Design review of the part built by this model. Coordinates are the model's own, in mm. Face numbers are marked on the shaded views. A direction names the side the tool comes from. Coordinates: 2 decimals unless noted, no trailing zeros. Order: outer loops, then holes, each group sorted by start corner. A loop starts at its lowest first (then second) coordinate and runs counter-clockwise, first axis right, second up. Notation, with made-up numbers: M -1.5,13 L 24.5,13 A30 cw 24.5,50 Z; hole C 22.25,37 d3. An arc over 180 degrees is marked long. Answer as a JSON object with one key per item and string values.
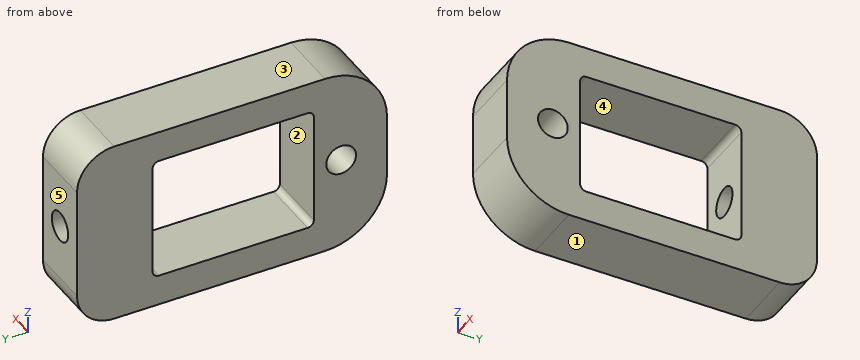
from build123d import *

# Parameters (mm, degrees)
SKETCH16_W                 = 5
SKETCH16_H                 = 15
MAIN_EXTRUDE_LOCKING_DEPTH = 25
SKETCH18_R                 = 1.2
CUT_EXTRUDE1_DEPTH         = 5
SKETCH8_W                  = 10
SKETCH8_H                  = 13
CUT_EXTRUDE2_DEPTH         = 5
SKETCH9_R                  = 1.2
CUT_EXTRUDE3_DEPTH         = 6.1
FILLET1_R                  = 5
FILLET2_R                  = 3
FILLET3_R                  = 0.5


with BuildPart() as part:
    # Sketch16 → Main Extrude_Locking (new body)
    with BuildSketch(Plane(origin=(0, 0, 0), x_dir=(1, 0, 0), z_dir=(0, 1, 0))):
        Rectangle(SKETCH16_W, SKETCH16_H)
    extrude(amount=MAIN_EXTRUDE_LOCKING_DEPTH)

    # Sketch18 → Cut-Extrude1 (cut)
    with BuildSketch(Plane.ZY.offset(2.5)):
        with Locations((0, 3.7)):
            Circle(SKETCH18_R)
    extrude(amount=-CUT_EXTRUDE1_DEPTH, mode=Mode.SUBTRACT)

    # Sketch8 → Cut-Extrude2 (cut)
    with BuildSketch(Plane.ZY.offset(2.5)):
        with Locations((0, 12.4)):
            Rectangle(SKETCH8_W, SKETCH8_H)
    extrude(amount=-CUT_EXTRUDE2_DEPTH, mode=Mode.SUBTRACT)

    # Sketch9 → Cut-Extrude3 (cut)
    with BuildSketch(Plane(origin=(0, 25, 0), x_dir=(1, 0, 0), z_dir=(0, 1, 0))):
        with Locations(Location((0, 0, 0), (0, 0, 270))):
            Circle(SKETCH9_R)
    extrude(amount=-CUT_EXTRUDE3_DEPTH, mode=Mode.SUBTRACT)

    # Fillet1
    fillet1_edges = [part.edges().sort_by_distance(p)[0] for p in [
        (0, 0, 7.5),
        (0, 0, -7.5),
    ]]
    fillet(fillet1_edges, radius=FILLET1_R)

    # Fillet2
    fillet2_edges = [part.edges().sort_by_distance(p)[0] for p in [
        (0, 25, 7.5),
        (0, 25, -7.5),
    ]]
    fillet(fillet2_edges, radius=FILLET2_R)

    # Fillet3
    fillet3_edges = [part.edges().sort_by_distance(p)[0] for p in [
        (0, 5.9, -5),
        (0, 18.9, -5),
        (0, 18.9, 5),
        (0, 5.9, 5),
    ]]
    fillet(fillet3_edges, radius=FILLET3_R)


solid = part.part
1) To check wall thickness, follow L1, parallel to Z at x = -0.1, y = 22; L2, parallel to Y at x = -0.2, z = 0; L3, parallel to Z at x = 2.1, y = 12.75. State the ranges of each line that lie inside material, in increasing order.
Taken from the geometry:
{"L1": "z = -7.5 to -1.2, 1.2 to 7.5", "L2": "y = 0 to 2.5, 4.9 to 5.9", "L3": "z = -7.5 to -5, 5 to 7.5"}
2) Add section A-A (y = 12). State the section outline as (x, z) points, and give its area (3 significant figures).
Taken from the geometry:
{"outline": "M -2.5,-7.5 L 2.5,-7.5 L 2.5,-5 L -2.5,-5 Z; M -2.5,5 L 2.5,5 L 2.5,7.5 L -2.5,7.5 Z", "area": "25.0 mm2"}
3) Add section C-C (x = 1.8). State the section outline as (y, z) points.
Taken from the geometry:
{"outline": "M 0,-2.5 A5 ccw 5,-7.5 L 22,-7.5 A3 ccw 25,-4.5 L 25,4.5 A3 ccw 22,7.5 L 5,7.5 A5 ccw 0,2.5 Z; hole C 3.7,0 d2.4; hole M 5.9,-4.5 A0.5 ccw 6.4,-5 L 18.4,-5 A0.5 ccw 18.9,-4.5 L 18.9,4.5 A0.5 ccw 18.4,5 L 6.4,5 A0.5 ccw 5.9,4.5 Z"}
4) Tool access review of the marked faces 4 and 5: name each direction out of +Z, -Z, +X, -X, +Y, -Y from which nothing blocks a thin tool from reaching the whole face with its end or side.
Taken from the geometry:
{"face 4": "+X, -X", "face 5": "+Z, -Z, +X, -X, +Y"}
5) Mouldability with a two-part tool opening along Z and no side actions: class the marked faces 1, 2 and 3 as released by +Z, released by -Z, zero draft, split by the parting line, or undercut.
Taken from the geometry:
{"face 1": "released by -Z", "face 2": "undercut", "face 3": "released by +Z"}
6) Add section B-B (z = 0). State the section outline as (x, y) points.
Taken from the geometry:
{"outline": "M -2.5,0 L 2.5,0 L 2.5,2.5 L -2.5,2.5 Z; M -2.5,4.9 L 2.5,4.9 L 2.5,5.9 L -2.5,5.9 Z; M -2.5,18.9 L -1.2,18.9 L -1.2,25 L -2.5,25 Z; M 1.2,18.9 L 2.5,18.9 L 2.5,25 L 1.2,25 Z"}
7) Add section D-D (x = 0). State the section outline as (y, z) points.
Taken from the geometry:
{"outline": "M 0,-2.5 A5 ccw 5,-7.5 L 22,-7.5 A3 ccw 25,-4.5 L 25,-1.2 L 18.9,-1.2 L 18.9,-4.5 A0.5 cw 18.4,-5 L 6.4,-5 A0.5 cw 5.9,-4.5 L 5.9,4.5 A0.5 cw 6.4,5 L 18.4,5 A0.5 cw 18.9,4.5 L 18.9,1.2 L 25,1.2 L 25,4.5 A3 ccw 22,7.5 L 5,7.5 A5 ccw 0,2.5 Z; hole C 3.7,0 d2.4"}
8) Insertion check: pin 1 Ø2 at (y, z) = (13.5, -4.5) entering from -X; pin 2 Ø1.9 at (y, z) = (3.7, 0) entering from +X. Each pin has a flat end and moves straight along its axis. Give the tip position at first contact, or say it passes through.
Taken from the geometry:
{"pin 1": "stops at x = -2.5", "pin 2": "passes through"}
